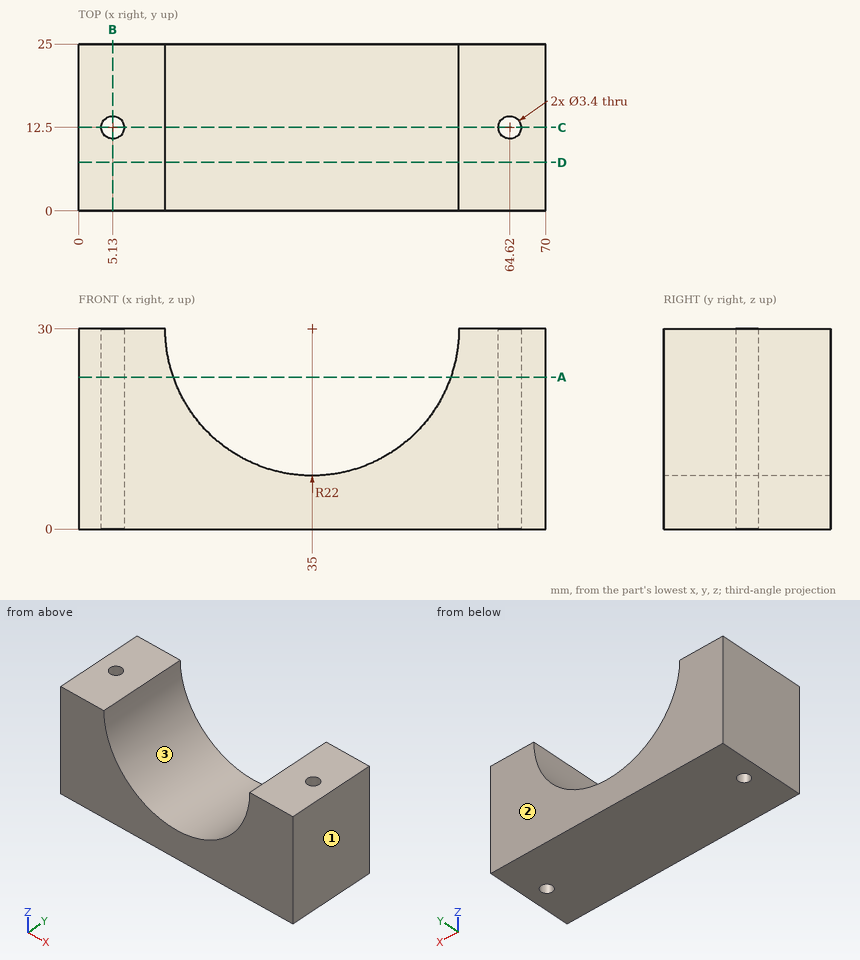
Job drawing, mm, ordinate dimensions from the low corner. One solid piece. Coordinates: 2 decimals unless noted, no trailing zeros. Order: outer loops, then holes, each group sorted by start corner. A loop starts at its lowest first (then second) coordinate and runs counter-clockwise, first axis right, second up. Notation, with made-up numbers: (-34.75, 51) -> (10.25, 51) arc R34 cw to (10.25, 87) -> close; hole circle Ø10 at (32.5, 64.25). An arc over 180 degrees is marked (long way). Return JSON: item names as keys, results as strings. Group by question number.
Item 1: Pull direction X, two halves, no side cores. Call the marked faces 1, 2 and 3: pulls with the +X half, pulls with the -X half, needs draft (parallel to the pull), parting line crosses it, or undercut.
Item 2: Saw through at B-B on x = 5.13. Write the cut outline in (y, z), then the cut area to 3 significant figures.
Item 3: Flat gauge pins, fed straight in: P1, Ø10, axis at x = 29, y = 10.5, coming from the +Z side; P2, Ø4, axis at x = 50.5, y = 3, coming from the +Z side; P3, Ø5.5, axis at x = 5.13, y = 12.5, coming from the -Z side. Where does each tip first touch, or does it go through?
Item 4: Wall check: line 1 along Y through (x, z) = (5.13, 21.25); line 2 along X through (y, z) = (17.25, 23.75); line 3 along X through (y, z) = (13.5, 12.75). Give the ranges that are in metal, low to high. Write a range as [from, to].
Item 5: Saw through at A-A on z = 22.75. Write the cut outline in (x, y), then the cut area to 3 significant figures.
Item 6: Saw through at D-D on y = 7.25. Write the cut outline in (x, z), then the cut area to 3 significant figures.
Item 7: Saw through at C-C on y = 12.5. Write the cut outline in (x, z), then the cut area to 3 significant figures.
Values found:
{
 "1": {"face 1": "pulls with the +X half", "face 2": "needs draft", "face 3": "undercut"},
 "2": {"outline": "(0, 0) -> (10.8, 0) -> (10.8, 30) -> (0, 30) -> close; (14.2, 0) -> (25, 0) -> (25, 30) -> (14.2, 30) -> close", "area": "648 mm2"},
 "3": {"P1": "stops at z = 10.95", "P2": "stops at z = 16.67", "P3": "stops at z = 0"},
 "4": {"line 1": "y = [0, 10.8], [14.2, 25]", "line 2": "x = [0, 13.91], [56.09, 70]", "line 3": "x = [0, 3.76], [6.5, 21.35], [48.65, 63.25], [65.99, 70]"},
 "5": {"outline": "(0, 0) -> (14.23, 0) -> (14.23, 25) -> (0, 25) -> close; (55.77, 0) -> (70, 0) -> (70, 25) -> (55.77, 25) -> close; hole circle Ø3.4 at (5.13, 12.5); hole circle Ø3.4 at (64.62, 12.5)", "area": "693 mm2"},
 "6": {"outline": "(0, 0) -> (70, 0) -> (70, 30) -> (57, 30) arc R22 cw to (13, 30) -> (0, 30) -> close", "area": "1,340 mm2"},
 "7": {"outline": "(0, 0) -> (3.43, 0) -> (3.43, 30) -> (0, 30) -> close; (6.83, 0) -> (62.92, 0) -> (62.92, 30) -> (57, 30) arc R22 cw to (13, 30) -> (6.83, 30) -> close; (66.32, 0) -> (70, 0) -> (70, 30) -> (66.32, 30) -> close", "area": "1,140 mm2"}
}
